Verification items for the finished model (mm, model axes). Face numbers are marked on the shaded views. A direction names the side the tool comes from. Coordinates: 2 decimals unless noted, no trailing zeros. Loops run counter-clockwise (first coordinate to the right, second up) from the corner with the lowest first, then second, coordinate; pieces in that order, holes last. Notation, with made-up numbers: (13.25, 57) - (18.25, 57) arc R23 ccw to (18.25, 89) - close; hole circle Ø10 at (82, -20). An arc over 180 degrees is marked (long way). One line per item, written item: value. Start each with the question number.
(1) Section check C-C (x = -2.75). Record the boundary of the cut face in (y, z).
(2) Gauge pin test, flat ends, axial feed: P1, Ø1.9, axis at x = 0, z = 0, coming from the +Y side; P2, Ø1.5, axis at y = 2.5, z = 5.5, coming from the +X side; P3, Ø4, axis at x = -3, y = 17, coming from the +Z side; P4, Ø6, axis at x = -5.5, y = 9.5, coming from the +Z side. Record the tip position at first contact, or that the pin passes through.
(3) Section check D-D (z = -5.25). Record the boundary of the cut face in (x, y).
(4) Draft check along X on the marked faces 3, 4 and 5. Enter one of: +X half, -X half, draft (parallel to the pull), parting line (faces both ways), or undercut.
(5) Section check B-B (y = 17.25). Record the boundary of the cut face in (x, z).
(6) Set-up check for the marked faces 1 and 2: record each of +Z, -Z, +X, -X, +Y, -Y from which the full face is reachable in a straight line by a thin tool's end or side.
(7) Thickness scan on probe 1 along X at (y, z) = (13.5, 0); probe 2 along X at (y, z) = (2, 0); probe 3 along Z at (x, y) = (1.25, 6.25). Record the ranges inside material, lowest first. Write a range as [from, to].
(8) Section check A-A (z = -1.25). Record the boundary of the cut face in (x, y).
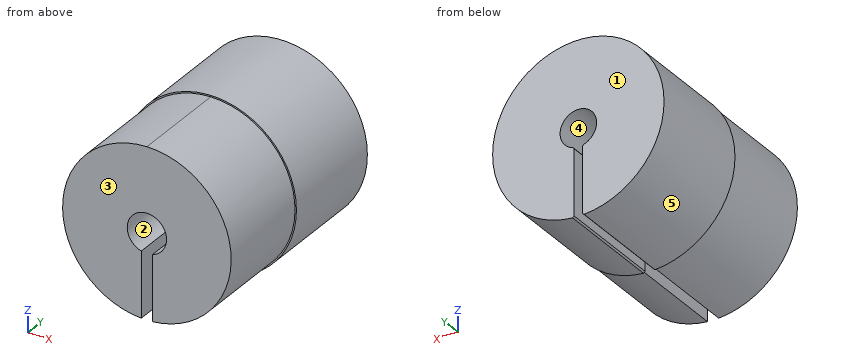
```python
from build123d import *

# Parameters (mm, degrees)
SKETCH1_R           = 7.5
BOSS_EXTRUDE1_DEPTH = 9
SKETCH2_R           = 1.75
CUT_EXTRUDE1_DEPTH  = 14.910427743
SKETCH4_W           = 1
SKETCH4_H           = 6.379821958
CUT_EXTRUDE2_DEPTH  = 9
BOSS_EXTRUDE2_DEPTH = 10


with BuildPart() as part:
    # Sketch1 → Boss-Extrude1 (new body)
    with BuildSketch(Plane(origin=(0, 0, 0), x_dir=(1, 0, 0), z_dir=(0, 1, 0))):
        with Locations(Location((0, 0, 0), (0, 0, 270))):
            Circle(SKETCH1_R)
    extrude(amount=BOSS_EXTRUDE1_DEPTH)

    # Sketch2 → Cut-Extrude1 (cut, through all)
    with BuildSketch(Plane(origin=(0, 9, 0), x_dir=(1, 0, 0), z_dir=(0, 1, 0))):
        with Locations(Location((0, 0, 0), (0, 0, 270))):
            Circle(SKETCH2_R)
    extrude(amount=-CUT_EXTRUDE1_DEPTH, mode=Mode.SUBTRACT)

    # Sketch4 → Cut-Extrude2 (cut)
    with BuildSketch(Plane(origin=(0, 9, 0), x_dir=(1, 0, 0), z_dir=(0, 1, 0))):
        with Locations((0, 4.574678536)):
            Rectangle(SKETCH4_W, SKETCH4_H)
    extrude(amount=-CUT_EXTRUDE2_DEPTH, mode=Mode.SUBTRACT)

    # Sketch5 → Boss-Extrude2 (add)
    # profile 1 of 2: a face of its own
    with BuildSketch(Plane(origin=(0, 9, 0), x_dir=(1, 0, 0), z_dir=(0, 1, 0))):
        with BuildLine():
            ThreePointArc((-0.463714286, 1.555344997), (0, -1.623), (0.463714286, 1.555344997))
            Line((0.463714286, 1.555344997), (0.373, 1.677050983))
            Line((0.373, 1.677050983), (0.373, 7.483314774))
            Line((0.373, 7.483314774), (0.508466667, 7.610032237))
            ThreePointArc((0.508466667, 7.610032237), (0, -7.627), (-0.508466667, 7.610032237))
            Line((-0.508466667, 7.610032237), (-0.373, 7.483314774))
            Line((-0.373, 7.483314774), (-0.373, 1.677050983))
            Line((-0.373, 1.677050983), (-0.463714286, 1.555344997))
        make_face()
        with BuildLine():
            Line((0.5, 7.483314774), (0.5, 1.677050983))
            ThreePointArc((0.5, 1.677050983), (0, -1.75), (-0.5, 1.677050983))
            Line((-0.5, 1.677050983), (-0.5, 7.483314774))
            ThreePointArc((-0.5, 7.483314774), (0, -7.5), (0.5, 7.483314774))
        make_face(mode=Mode.SUBTRACT)
    # profile 2 of 2: a face of its own
    with BuildSketch(Plane(origin=(0, 9, 0), x_dir=(1, 0, 0), z_dir=(0, 1, 0))):
        with BuildLine():
            ThreePointArc((-0.5, 7.483314774), (0, -7.5), (0.5, 7.483314774))
            Line((0.5, 7.483314774), (0.5, 1.677050983))
            ThreePointArc((0.5, 1.677050983), (0, -1.75), (-0.5, 1.677050983))
            Line((-0.5, 1.677050983), (-0.5, 7.483314774))
        make_face()
    extrude(amount=BOSS_EXTRUDE2_DEPTH)


solid = part.part
```
Responses:
1. outline: (0, -6.98) - (9, -6.98) - (9, -7.11) - (19, -7.11) - (19, 7.11) - (9, 7.11) - (9, 6.98) - (0, 6.98) - close
2. P1: passes through
2. P2: stops at x = 5.8
2. P3: stops at z = 7.56
2. P4: stops at z = 7.21
3. outline: (-5.53, 9) - (-5.36, 9) - (-5.36, 0) - (-0.5, 0) - (-0.5, 9) - (-0.37, 9) - (-0.37, 19) - (-5.53, 19) - close; (0.37, 9) - (0.5, 9) - (0.5, 0) - (5.36, 0) - (5.36, 9) - (5.53, 9) - (5.53, 19) - (0.37, 19) - close
4. face 3: draft
4. face 4: undercut
4. face 5: parting line
5. outline: (-0.51, -7.61) - (-0.37, -7.48) - (-0.37, -1.68) - (-0.46, -1.56) arc R1.62 cw (long way) to (0.46, -1.56) - (0.37, -1.68) - (0.37, -7.48) - (0.51, -7.61) arc R7.63 ccw (long way) to start
6. face 1: +Z, -Z, +X, -X, +Y
6. face 2: -Y
7. probe 1: x = [-7.63, -1.62], [1.62, 7.63]
7. probe 2: x = [-7.5, -1.75], [1.75, 7.5]
7. probe 3: z = [-7.4, -1.22], [1.22, 7.4]
8. outline: (-7.52, 9) - (-7.4, 9) - (-7.4, 0) - (-1.22, 0) - (-1.22, 9) - (-1.04, 9) - (-1.04, 19) - (-7.52, 19) - close; (1.04, 9) - (1.22, 9) - (1.22, 0) - (7.4, 0) - (7.4, 9) - (7.52, 9) - (7.52, 19) - (1.04, 19) - close
